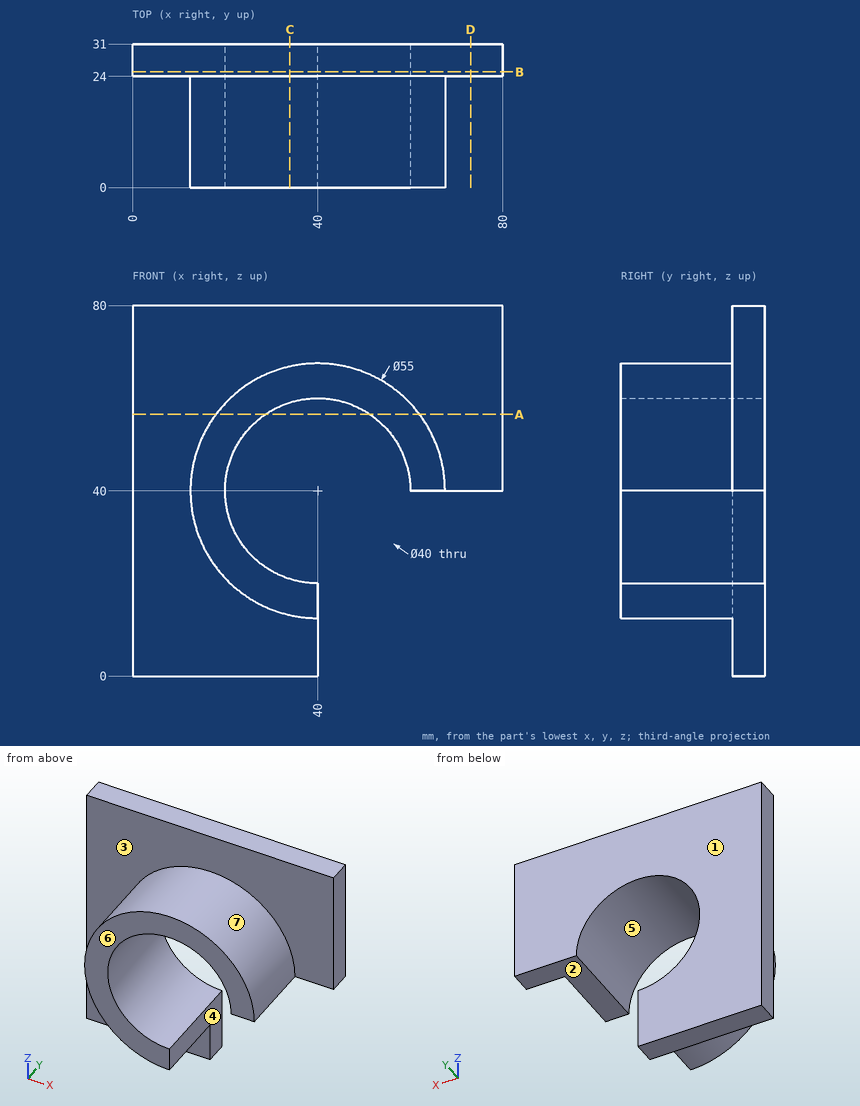
Geometry check sheet. Reference: drawing and pictorial views, mm from the part's lowest x, y, z. A direction names the side the tool comes from. Give positions to 0.01 mm unless a question says otherwise; leave off trailing zeros. Order: outer loops, then holes, each group sorted by start corner. A loop starts at its lowest first (then second) coordinate and runs counter-clockwise, first axis right, second up. Notation, with made-up numbers: (14.5, 37.25) -> (41.5, 37.25) arc R29 cw to (41.5, 67.25) -> close; hole circle Ø2 at (-26, 43.5). An arc over 180 degrees is marked (long way). Write each question's results on one line, items separated by ' | '. Start each with the question number.
(1) Gauge pin test, flat ends, axial feed: P1, Ø10, axis at x = 69, y = 23, coming from the -Z side; P2, Ø24, axis at x = 40, z = 40, coming from the +Y side; P3, Ø5, axis at y = 25, z = 30, coming from the +X side; P4, Ø1.5, axis at y = 21, z = 48.5, coming from the +X side. Record the tip position at first contact, or that the pin passes through.
(2) Sectioned sample at C-C (x = 34). Enter the section's corners in (y, z).
(3) Access from +Z, -Z, +X, -X, +Y, -Y to the whole of each face (thin tool, end or side, straight path). Record for the marked faces 1, 2 and 3.
(4) Mould release check, pull along X, two halves, no side actions. Record for the marked faces 4, 5, 6 and 7: pulls with the +X half, pulls with the -X half, needs draft (parallel to the pull), parting line crosses it, or undercut.
(5) Sectioned sample at A-A (z = 56.5). Enter the section's corners in (x, y).
(6) Sectioned sample at B-B (y = 25). Enter the section's corners in (x, z), plus the area to 3 significant figures.
(7) Scan lines: line 1 (X direction, y = 27, z = 8.5); line 2 (Y direction, x = 13.5, z = 70); line 3 (X direction, y = 21.5, z = 51.5). Record each from-to range of solid material in increasing order.
(8) Sectioned sample at D-D (x = 73). Enter the section's corners in (y, z).
Answer below:
1) P1: z = 40 | P2: through | P3: x = 24.39 | P4: x = 66.39
2) outline: (0, 13.16) -> (24, 13.16) -> (24, 0) -> (31, 0) -> (31, 20.92) -> (0, 20.92) -> close; (0, 59.08) -> (31, 59.08) -> (31, 80) -> (24, 80) -> (24, 66.84) -> (0, 66.84) -> close
3) face 1: +Z, -Z, +X, -X, +Y | face 2: -Z, +X, +Y, -Y | face 3: -Y
4) face 4: pulls with the +X half | face 5: undercut | face 6: needs draft | face 7: parting line crosses it
5) outline: (0, 24) -> (18, 24) -> (18, 0) -> (28.7, 0) -> (28.7, 31) -> (0, 31) -> close; (51.3, 0) -> (62, 0) -> (62, 24) -> (80, 24) -> (80, 31) -> (51.3, 31) -> close
6) outline: (0, 0) -> (40, 0) -> (40, 20) arc R20 cw (long way) to (60, 40) -> (80, 40) -> (80, 80) -> (0, 80) -> close | area: 3,860 mm2
7) line 1: 0 to 40 | line 2: 24 to 31 | line 3: 15.02 to 23.64, 56.36 to 64.98
8) outline: (24, 40) -> (31, 40) -> (31, 80) -> (24, 80) -> close
